```python
from build123d import *

# Parameters (mm, degrees)
SKETCH1_W                = 12.409227922
SKETCH1_H                = 25.738488059
SKETCH1_R                = 1
SKETCH1_W_2              = 8.15
SKETCH1_H_2              = 18.7
BOSS_EXTRUDE1_DEPTH      = 3
SKETCH15_W               = 27.240995133
SKETCH15_H               = 25.738488059
BOSS_EXTRUDE5_DEPTH      = 4
SKETCH16_R               = 3.1
CUT_EXTRUDE12_DEPTH      = 1.5
CUT_EXTRUDE13_DEPTH      = 1.2
CHAMFER1_SIZE            = 2
CUT_EXTRUDE14_DEPTH      = 31.943326143
CUT_EXTRUDE14_DEPTH_BACK = 31.943326143
SKETCH18_R               = 1.5
SKETCH18_R_2             = 0.5
FILLET1_R                = 3
FILLET2_R                = 3
BOSS_EXTRUDE7_DEPTH      = 5
CUT_EXTRUDE15_DEPTH      = 39.151604311
CUT_EXTRUDE15_DEPTH_BACK = 39.151604311
CHAMFER2_SIZE            = 3
SKETCH23_R               = 3.318889956
SKETCH23_R_2             = 1.409018686
CUT_EXTRUDE17_DEPTH      = 1
FILLET4_R                = 3
BOSS_EXTRUDE8_DEPTH      = 12.409227923
SKETCH25_R               = 1.5
CUT_EXTRUDE18_DEPTH      = 13
SKETCH26_R               = 2.992034133
CUT_EXTRUDE19_DEPTH      = 1
FILLET5_SIZE             = 8
FILLET6_R                = 4
SKETCH27_W               = 9.781799862
SKETCH27_H               = 23.423713079
CUT_EXTRUDE20_DEPTH      = 1.5
FILLET7_R                = 2


with BuildPart() as part:
    # Sketch1 → Boss-Extrude1 (new body)
    with BuildSketch(Plane(origin=(0, 0, 0), x_dir=(0, 0, -1), z_dir=(1, 0, 0))):
        with Locations((1.233520205, 9.896555647)):
            Rectangle(SKETCH1_W, SKETCH1_H)
        with Locations((1.233520205, 20.798227972)):
            Circle(SKETCH1_R, mode=Mode.SUBTRACT)
        with Locations((1.233520205, -1.111772028)):
            Circle(SKETCH1_R, mode=Mode.SUBTRACT)
        with Locations((1.233520205, 9.843227972)):
            Rectangle(SKETCH1_W_2, SKETCH1_H_2, mode=Mode.SUBTRACT)
    extrude(amount=BOSS_EXTRUDE1_DEPTH)

    # Sketch15 → Boss-Extrude5 (add)
    with BuildSketch(Plane.XY.offset(4.971093756)):
        with Locations((-1.10779903, 9.896555647)):
            Rectangle(SKETCH15_W, SKETCH15_H)
    extrude(amount=BOSS_EXTRUDE5_DEPTH)

    # Sketch16 → Cut-Extrude12 (cut)
    with BuildSketch(Plane.XY.offset(8.971093756)):
        with Locations((-6.437606402, 10.038669905)):
            Circle(SKETCH16_R)
    extrude(amount=-CUT_EXTRUDE12_DEPTH, mode=Mode.SUBTRACT)

    # Sketch17 → Cut-Extrude13 (cut)
    with BuildSketch(Plane.XY.offset(8.971093756)):
        Polygon((-6.437606402, 10.038669905), (-8.187606402, 10.038669905), (-8.187606402, 0.412009525), (-4.687606402, 0.412009525), (-4.687606402, 10.038669905), align=None)
    extrude(amount=-CUT_EXTRUDE13_DEPTH, mode=Mode.SUBTRACT)

    # Chamfer1
    chamfer1_edges = [part.edges().sort_by_distance(p)[0] for p in [
        (-14.728296596, 22.765799677, 6.971093756),
        (-14.728296596, -2.972688382, 6.971093756),
        (12.512698537, -2.972688382, 6.971093756),
        (12.512698537, 22.765799677, 6.971093756),
    ]]
    chamfer(chamfer1_edges, length=CHAMFER1_SIZE)

    # Sketch18 → Cut-Extrude14 (cut, two sides: drawn at the far end of the back side and taken through both)
    with BuildSketch(Plane.XY.offset(7.471093756).offset(-CUT_EXTRUDE14_DEPTH_BACK)):
        with Locations((-6.437606402, 10.038669905)):
            Circle(SKETCH18_R)
        with Locations((-6.437606402, 2.038669905)):
            Circle(SKETCH18_R_2)
    extrude(amount=CUT_EXTRUDE14_DEPTH + CUT_EXTRUDE14_DEPTH_BACK, mode=Mode.SUBTRACT)

    # Fillet1
    fillet1_edges = [part.edges().sort_by_distance(p)[0] for p in [
        (1.5, -2.972688382, -7.438134166),
        (1.5, 22.765799677, -7.438134166),
    ]]
    fillet(fillet1_edges, radius=FILLET1_R)

    # Fillet2
    # the kernel refuses this fillet: 3 mm, written as the material it adds along each edge
    with BuildSketch(Plane(origin=(3, -2.972688382, 4.971093756), x_dir=(0, 0, -1), z_dir=(0, 1, 0))) as fillet2_piece_1_section:
        with BuildLine():
            CenterArc((FILLET2_R, -FILLET2_R), FILLET2_R, 90, 90)
            Line((0, -FILLET2_R), (0, 0))
            Line((0, 0), (FILLET2_R, 0))
        make_face()
    fillet2_piece_1 = extrude(amount=25.738488059, mode=Mode.PRIVATE)
    fillet2_piece_1 = split(fillet2_piece_1, bisect_by=Plane(origin=(3, -2.972688382, 2.841479795), z_dir=(0, 0, -1)), keep=Keep.TOP, mode=Mode.PRIVATE)
    fillet2_piece_1 = split(fillet2_piece_1, bisect_by=Plane(origin=(3, 0.493227972, 4.971093756), z_dir=(0, -1, 0)), keep=Keep.TOP, mode=Mode.PRIVATE)
    add(fillet2_piece_1)
    with BuildSketch(Plane(origin=(3, -2.972688382, 4.971093756), x_dir=(0, 0, -1), z_dir=(0, 1, 0))) as fillet2_piece_2_section:
        with BuildLine():
            CenterArc((FILLET2_R, -FILLET2_R), FILLET2_R, 90, 90)
            Line((0, -FILLET2_R), (0, 0))
            Line((0, 0), (FILLET2_R, 0))
        make_face()
    fillet2_piece_2 = extrude(amount=25.738488059, mode=Mode.PRIVATE)
    fillet2_piece_2 = split(fillet2_piece_2, bisect_by=Plane(origin=(3, -2.972688382, 2.841479795), z_dir=(0, 0, 1)), keep=Keep.TOP, mode=Mode.PRIVATE)
    fillet2_piece_2 = split(fillet2_piece_2, bisect_by=Plane(origin=(3, 0.493227972, 4.971093756), z_dir=(0, -1, 0)), keep=Keep.TOP, mode=Mode.PRIVATE)
    add(fillet2_piece_2)
    with BuildSketch(Plane(origin=(3, -2.972688382, 4.971093756), x_dir=(0, 0, -1), z_dir=(0, 1, 0))) as fillet2_piece_3_section:
        with BuildLine():
            CenterArc((FILLET2_R, -FILLET2_R), FILLET2_R, 90, 90)
            Line((0, -FILLET2_R), (0, 0))
            Line((0, 0), (FILLET2_R, 0))
        make_face()
    fillet2_piece_3 = extrude(amount=25.738488059, mode=Mode.PRIVATE)
    fillet2_piece_3 = split(fillet2_piece_3, bisect_by=Plane(origin=(3, 19.193227972, 4.971093756), z_dir=(0, -1, 0)), keep=Keep.TOP, mode=Mode.PRIVATE)
    fillet2_piece_3 = split(fillet2_piece_3, bisect_by=Plane(origin=(3, -2.972688382, 2.841479795), z_dir=(0, 0, 1)), keep=Keep.TOP, mode=Mode.PRIVATE)
    fillet2_piece_3 = split(fillet2_piece_3, bisect_by=Plane(origin=(3, 0.493227972, 4.971093756), z_dir=(0, 1, 0)), keep=Keep.TOP, mode=Mode.PRIVATE)
    add(fillet2_piece_3)
    with BuildSketch(Plane(origin=(3, -2.972688382, 4.971093756), x_dir=(0, 0, -1), z_dir=(0, 1, 0))) as fillet2_piece_4_section:
        with BuildLine():
            CenterArc((FILLET2_R, -FILLET2_R), FILLET2_R, 90, 90)
            Line((0, -FILLET2_R), (0, 0))
            Line((0, 0), (FILLET2_R, 0))
        make_face()
    fillet2_piece_4 = extrude(amount=25.738488059, mode=Mode.PRIVATE)
    fillet2_piece_4 = split(fillet2_piece_4, bisect_by=Plane(origin=(3, 19.193227972, 4.971093756), z_dir=(0, 1, 0)), keep=Keep.TOP, mode=Mode.PRIVATE)
    fillet2_piece_4 = split(fillet2_piece_4, bisect_by=Plane(origin=(3, -2.972688382, 2.841479795), z_dir=(0, 0, -1)), keep=Keep.TOP, mode=Mode.PRIVATE)
    add(fillet2_piece_4)
    with BuildSketch(Plane(origin=(3, -2.972688382, 4.971093756), x_dir=(0, 0, -1), z_dir=(0, 1, 0))) as fillet2_piece_5_section:
        with BuildLine():
            CenterArc((FILLET2_R, -FILLET2_R), FILLET2_R, 90, 90)
            Line((0, -FILLET2_R), (0, 0))
            Line((0, 0), (FILLET2_R, 0))
        make_face()
    fillet2_piece_5 = extrude(amount=25.738488059, mode=Mode.PRIVATE)
    fillet2_piece_5 = split(fillet2_piece_5, bisect_by=Plane(origin=(3, 19.193227972, 4.971093756), z_dir=(0, 1, 0)), keep=Keep.TOP, mode=Mode.PRIVATE)
    fillet2_piece_5 = split(fillet2_piece_5, bisect_by=Plane(origin=(3, -2.972688382, 2.841479795), z_dir=(0, 0, 1)), keep=Keep.TOP, mode=Mode.PRIVATE)
    add(fillet2_piece_5)

    # Sketch20 → Boss-Extrude7 (add)
    with BuildSketch(Plane.XY.offset(8.971093756)):
        Polygon((-12.728296596, 22.765799677), (-14.728296596, 20.765799677), (-14.728296596, -0.972688382), (-12.728296596, -2.972688382), (10.512698537, -2.972688382), (12.512698537, -0.972688382), (12.512698537, 20.765799677), (10.512698537, 22.765799677), align=None)
        Polygon((9.145793781, 0.327311618), (9.212698537, 0.394216374), (9.212698537, 19.398894921), (9.145793781, 19.465799677), (-11.36139184, 19.465799677), (-11.428296596, 19.398894921), (-11.428296596, 0.394216374), (-11.36139184, 0.327311618), align=None, mode=Mode.SUBTRACT)
    extrude(amount=BOSS_EXTRUDE7_DEPTH)

    # Sketch21 → Cut-Extrude15 (cut, two sides: drawn at the far end of the back side and taken through both)
    with BuildSketch(Plane.ZY.offset(14.728296596).offset(-CUT_EXTRUDE15_DEPTH_BACK)):
        Polygon((0.508600598, 22.765799677), (13.971093756, 19.274181739), (13.971093756, 24.16200456), (0.508600598, 24.16200456), align=None)
        Polygon((0.508600598, -4.368893265), (0.508600598, -2.972688382), (13.971093756, 0.518929556), (13.971093756, -4.368893265), align=None)
    extrude(amount=CUT_EXTRUDE15_DEPTH + CUT_EXTRUDE15_DEPTH_BACK, mode=Mode.SUBTRACT)

    # Chamfer2
    chamfer2_edges = [part.edges().sort_by_distance(p)[0] for p in [
        (-14.728296596, -0.226879413, 11.095507618),
        (12.512698537, 20.019990708, 11.095507618),
        (12.512698537, -0.226879413, 11.095507618),
        (-14.728296596, 20.019990708, 11.095507618),
    ]]
    chamfer(chamfer2_edges, length=CHAMFER2_SIZE)

    # Sketch23 → Cut-Extrude17 (cut)
    with BuildSketch(Plane(origin=(0, 0, 4.971093756), x_dir=(-1, 0, 0), z_dir=(0, 0, -1))):
        with Locations((6.437606402, 10.038669905)):
            Circle(SKETCH23_R)
        with Locations((6.437606402, 2.038669905)):
            Circle(SKETCH23_R_2)
    extrude(amount=-CUT_EXTRUDE17_DEPTH, mode=Mode.SUBTRACT)

    # Fillet4
    # the kernel refuses this fillet: 3 mm, written as the material it adds along each edge
    with BuildSketch(Plane(origin=(9.212698537, -7.105783626, 8.971093756), x_dir=(0, 0, 1), z_dir=(0, 1, 0))) as fillet4_piece_1_section:
        with BuildLine():
            CenterArc((FILLET4_R, -FILLET4_R), FILLET4_R, 90, 90)
            Line((0, -FILLET4_R), (0, 0))
            Line((0, 0), (FILLET4_R, 0))
        make_face()
    fillet4_piece_1 = extrude(amount=34.004678547, mode=Mode.PRIVATE)
    fillet4_piece_1 = split(fillet4_piece_1, bisect_by=Plane(origin=(9.212698537, 19.465799677, 8.971093756), z_dir=(0, -1, 0)), keep=Keep.TOP, mode=Mode.PRIVATE)
    fillet4_piece_1 = split(fillet4_piece_1, bisect_by=Plane(origin=(9.212698537, 0.327311618, 8.971093756), z_dir=(0, 1, 0)), keep=Keep.TOP, mode=Mode.PRIVATE)
    add(fillet4_piece_1)
    with BuildSketch(Plane(origin=(16.645793781, 19.465799677, 8.971093756), x_dir=(0, 0, 1), z_dir=(-1, 0, 0))) as fillet4_piece_2_section:
        with BuildLine():
            CenterArc((FILLET4_R, -FILLET4_R), FILLET4_R, 90, 90)
            Line((0, -FILLET4_R), (0, 0))
            Line((0, 0), (FILLET4_R, 0))
        make_face()
    fillet4_piece_2 = extrude(amount=35.50718562, mode=Mode.PRIVATE)
    fillet4_piece_2 = split(fillet4_piece_2, bisect_by=Plane(origin=(12.895793781, 15.715799677, 8.971093756), z_dir=(-0.707106781186557, -0.7071067811865381, 0)), keep=Keep.TOP, mode=Mode.PRIVATE)
    fillet4_piece_2 = split(fillet4_piece_2, bisect_by=Plane(origin=(-11.428296596, 19.465799677, 8.971093756), z_dir=(1, 0, 0)), keep=Keep.TOP, mode=Mode.PRIVATE)
    add(fillet4_piece_2)

    # Sketch24 → Boss-Extrude8 (add)
    with BuildSketch(Plane(origin=(0, 0, 4.971093756), x_dir=(-1, 0, 0), z_dir=(0, 0, -1))):
        Polygon((14.728296596, 8.32475399), (9.781799862, 8.32475399), (9.781799862, -1.815300892), (11.728296596, -1.815300892), (14.728296596, 1.283957653), align=None)
    extrude(amount=BOSS_EXTRUDE8_DEPTH)

    # Sketch25 → Cut-Extrude18 (cut)
    with BuildSketch(Plane.ZY.offset(14.728296596)):
        with Locations((-1.233520205, 4.70072857)):
            Circle(SKETCH25_R)
    extrude(amount=-CUT_EXTRUDE18_DEPTH, mode=Mode.SUBTRACT)

    # Sketch26 → Cut-Extrude19 (cut)
    with BuildSketch(Plane.ZY.offset(14.728296596)):
        with Locations((-1.233520205, 4.70072857)):
            Circle(SKETCH26_R)
    extrude(amount=-CUT_EXTRUDE19_DEPTH, mode=Mode.SUBTRACT)

    # Fillet5
    # a fillet whose section is not a circle: 8 mm, written as the material it adds along each edge
    with BuildSketch(Plane(origin=(-14.728296596, 8.32475399, 4.971093756), x_dir=(0, 1, 0), z_dir=(1, 0, 0))) as fillet5_piece_1:
        with BuildLine():
            Bezier((FILLET5_SIZE, 0), (0, 0), (0, -FILLET5_SIZE), weights=[1, 0.538461538, 1])
            Line((0, -FILLET5_SIZE), (0, 0))
            Line((0, 0), (FILLET5_SIZE, 0))
        make_face()
    extrude(amount=4.946496733)

    # Fillet6
    fillet6_edges = [part.edges().sort_by_distance(p)[0] for p in [
        (-10.755048229, -1.815300892, -7.438134167),
    ]]
    fillet(fillet6_edges, radius=FILLET6_R)

    # Sketch27 → Cut-Extrude20 (cut)
    with BuildSketch(Plane(origin=(0, 0, 4.971093756), x_dir=(-1, 0, 0), z_dir=(0, 0, -1))):
        with Locations((4.890899931, 9.896555648)):
            Rectangle(SKETCH27_W, SKETCH27_H)
    extrude(amount=-CUT_EXTRUDE20_DEPTH, mode=Mode.SUBTRACT)

    # Fillet7
    fillet7_edges = [part.edges().sort_by_distance(p)[0] for p in [
        (0, 9.896555648, 6.471093756),
    ]]
    fillet(fillet7_edges, radius=FILLET7_R)


solid = part.part
```
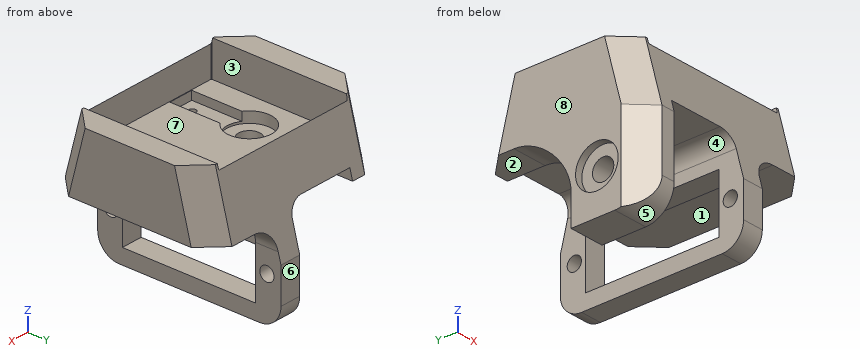
Work out the finished part from the listing and answer in its coordinate system (mm). Face numbers are marked on the shaded views. A direction names the side the tool comes from. Coordinates: 2 decimals unless noted, no trailing zeros. Loops run counter-clockwise (first coordinate to the right, second up) from the corner with the lowest first, then second, coordinate; pieces in that order, holes last. Notation, with made-up numbers: (88.5, -28.75) - (110.5, -28.75) arc R24 ccw to (110.5, 4.25) - close; hole circle Ø5 at (87.25, 28.25). An arc over 180 degrees is marked (long way). Use a Markdown table: item, result.
Item 1: Consider probe 1 along Z at (x, y) = (1.75, 7); probe 2 along X at (y, z) = (8.75, 13); probe 3 along Z at (x, y) = (6.25, 10). Determine where each line is inside the solid, lowest interval first. Write a range as from..to.
Evaluation:
| item | result |
|---|---|
| probe 1 | z = -7.44..-5.31, 2.84..8.97 |
| probe 2 | x = -14.73..-11.43, 9.21..12.51 |
| probe 3 | z = 4.97..8.97 |
Item 2: Find section A-A, the plane z = 5.5. Determine the outline of the cut face in (x, y).
Evaluation:
| item | result |
|---|---|
| outline | (-14.73, 1.42) - (-11.73, -1.68) - (-9.78, -1.68) - (-9.78, 21.47) - (-11.73, 21.47) - (-14.73, 18.37) - close; (-0.28, -1.68) - (9.51, -1.68) - (12.51, 1.42) - (12.51, 18.37) - (9.51, 21.47) - (-0.28, 21.47) - close |
Item 3: The mould has two halves that part along Y. Classify the marked faces 6, 7 and 8: +Y half, -Y half, draft (parallel to the pull), parting line (faces both ways), or undercut.
Evaluation:
| item | result |
|---|---|
| face 6 | +Y half |
| face 7 | undercut |
| face 8 | draft |
Item 4: Find section B-B, the plane y = 17. Determine the outline of the cut face in (x, z).
Evaluation:
| item | result |
|---|---|
| outline | (-14.73, 4.97) - (-9.78, 4.97) - (-9.78, 6.47) - (-2, 6.47) arc R2 cw to (0, 4.47) - (0, 2.84) - (3.13, 2.84) arc R3 cw to (6, 4.97) - (12.51, 4.97) - (12.51, 10.79) - (11.71, 13.97) - (9.21, 13.97) - (9.21, 11.97) arc R3 cw to (6.75, 9.02) - (-11.43, 9.02) - (-11.43, 13.97) - (-13.93, 13.97) - (-14.73, 10.79) - close; (0, -7.44) - (3, -7.44) - (3, -5.31) - (0, -5.31) - close |
Item 5: Find section D-D, the plane z = 12.75. Determine the outline of the cut face in (x, y).
Evaluation:
| item | result |
|---|---|
| outline | (-14.73, 3.3) - (-11.73, 0.2) - (9.51, 0.2) - (12.51, 3.3) - (12.51, 16.49) - (9.51, 19.59) - (-11.73, 19.59) - (-14.73, 16.49) - close; hole (-11.43, 0.39) - (-11.36, 0.33) - (9.15, 0.33) - (9.21, 0.39) - (9.21, 19.4) - (9.15, 19.47) - (-11.36, 19.47) - (-11.43, 19.4) - close |
Item 6: Given pin 1 Ø6 at (x, z) = (-9, 2.5) entering from +Y; pin 2 Ø4 at (x, y) = (-6.5, 7) entering from -Z; pin 3 Ø2.5 at (x, y) = (-6.44, 10.04) entering from -Z; pin 4 Ø2.5 at (y, z) = (20.8, -1.23) entering from -X, each flat-ended and moving along its own axis, determine where each tip first touches the part or whether it passes through.
Evaluation:
| item | result |
|---|---|
| pin 1 | stops at y = 21.61 |
| pin 2 | stops at z = 6.47 |
| pin 3 | passes through |
| pin 4 | stops at x = 0 |
Item 7: For the marked faces 1, 2, 3, 4 and 5, determine the directions among +Z, -Z, +X, -X, +Y, -Y from which every point of the face is accessible in a straight line to the end or side of a thin tool.
Evaluation:
| item | result |
|---|---|
| face 1 | -Z, +X, +Y, -Y |
| face 2 | -Z, -X, +Y |
| face 3 | +Z |
| face 4 | -Z, +Y, -Y |
| face 5 | -Z, -X, -Y |
Item 8: Find section C-C, the plane x = 1.75. Determine the outline of the cut face in (y, z).
Evaluation:
| item | result |
|---|---|
| outline | (-2.97, -4.44) arc R3 ccw to (0.03, -7.44) - (19.77, -7.44) arc R3 ccw to (22.77, -4.44) - (22.77, 0.51) - (19.47, 13.23) - (19.47, 11.97) arc R3 cw to (16.47, 8.97) - (0.33, 8.97) - (0.33, 13.23) - (-2.97, 0.51) - close; hole circle Ø2 at (-1.11, -1.23); hole (0.49, -5.31) - (19.19, -5.31) - (19.19, 2.84) - (0.49, 2.84) - close; hole circle Ø2 at (20.8, -1.23) |
